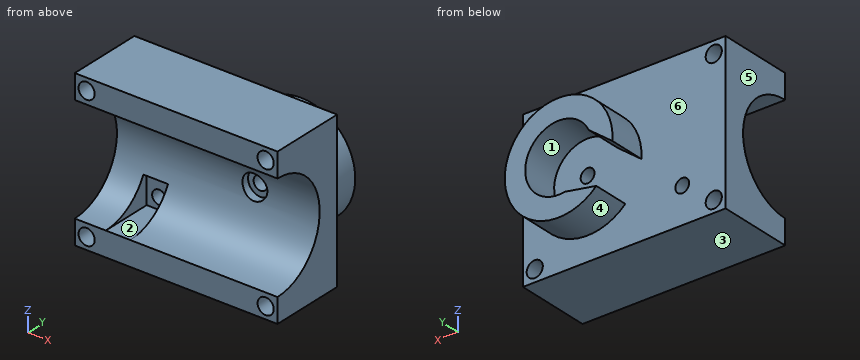
```python
from build123d import *

# Parameters (mm, degrees)
SKETCH1_W           = 60
SKETCH1_H           = 36
BOSS_EXTRUDE1_DEPTH = 35
SKETCH3_R           = 12.375
CUT_EXTRUDE1_DEPTH  = 61
SKETCH5_R           = 1.875
CUT_EXTRUDE2_DEPTH  = 40
CUT_EXTRUDE3_START  = 30
SKETCH7_W           = 36
SKETCH7_H           = 17.5
CUT_EXTRUDE3_DEPTH  = 61
SKETCH19_R          = 2.885
CUT_EXTRUDE13_DEPTH = 14
SKETCH20_R          = 1.6
CUT_EXTRUDE14_DEPTH = 13
SKETCH21_R          = 1.6
CUT_EXTRUDE15_DEPTH = 18.5000001
SKETCH22_W          = 5.7
SKETCH22_H          = 6.805143355
CUT_EXTRUDE16_DEPTH = 12
SKETCH23_R          = 12.5
SKETCH23_R_2        = 7.75
BOSS_EXTRUDE2_DEPTH = 8.5
CUT_EXTRUDE17_DEPTH = 8.5
SKETCH25_W          = 40.384912637
SKETCH25_H          = 20.483413903
CUT_EXTRUDE18_DEPTH = 13


with BuildPart() as part:
    # Sketch1 → Boss-Extrude1 (new body)
    with BuildSketch(Plane(origin=(0, 0, 0), x_dir=(1, 0, 0), z_dir=(0, 1, 0))):
        Rectangle(SKETCH1_W, SKETCH1_H)
    extrude(amount=BOSS_EXTRUDE1_DEPTH)

    # Sketch3 → Cut-Extrude1 (cut, through all)
    with BuildSketch(Plane(origin=(30, 0, 0), x_dir=(0, 0, -1), z_dir=(1, 0, 0))):
        with Locations((0, 17.5)):
            Circle(SKETCH3_R)
    extrude(amount=-CUT_EXTRUDE1_DEPTH, mode=Mode.SUBTRACT)

    # Sketch5 → Cut-Extrude2 (cut)
    with BuildSketch(Plane(origin=(0, 35, 0), x_dir=(1, 0, 0), z_dir=(0, 1, 0))):
        with Locations((27.25, -15.25)):
            Circle(SKETCH5_R)
        with Locations((27.25, 15.25)):
            Circle(SKETCH5_R)
        with Locations((-14.25, -15.25)):
            Circle(SKETCH5_R)
        with Locations((-14.25, 15.25)):
            Circle(SKETCH5_R)
    extrude(amount=-CUT_EXTRUDE2_DEPTH, mode=Mode.SUBTRACT)

    # Sketch7 → Cut-Extrude3 (cut, through all)
    with BuildSketch(Plane(origin=(0, 0, 0), x_dir=(0, 0, -1), z_dir=(1, 0, 0)).offset(CUT_EXTRUDE3_START)):
        with Locations((0, 8.75)):
            Rectangle(SKETCH7_W, SKETCH7_H)
    extrude(amount=-CUT_EXTRUDE3_DEPTH, mode=Mode.SUBTRACT)

    # Sketch19 → Cut-Extrude13 (cut)
    with BuildSketch(Plane.XZ.offset(-17.5)):
        with Locations((15, 0)):
            Circle(SKETCH19_R)
    extrude(amount=-CUT_EXTRUDE13_DEPTH, mode=Mode.SUBTRACT)

    # Sketch20 → Cut-Extrude14 (cut)
    with BuildSketch(Plane.XZ.offset(-31.5)):
        with Locations((15, 0)):
            Circle(SKETCH20_R)
    extrude(amount=-CUT_EXTRUDE14_DEPTH, mode=Mode.SUBTRACT)

    # Sketch21 → Cut-Extrude15 (cut, through all)
    with BuildSketch(Plane(origin=(0, 35, 0), x_dir=(1, 0, 0), z_dir=(0, 1, 0))):
        with Locations((-6.937800687, 9.733082811)):
            Circle(SKETCH21_R)
    extrude(amount=-CUT_EXTRUDE15_DEPTH, mode=Mode.SUBTRACT)

    # Sketch22 → Cut-Extrude16 (cut)
    with BuildSketch(Plane.XZ.offset(-17.5)):
        with Locations((-6.954606202, -8.972428323)):
            Rectangle(SKETCH22_W, SKETCH22_H)
    extrude(amount=-CUT_EXTRUDE16_DEPTH, mode=Mode.SUBTRACT)

    # Sketch23 → Boss-Extrude2 (add)
    with BuildSketch(Plane(origin=(0, 35, 0), x_dir=(1, 0, 0), z_dir=(0, 1, 0))):
        with Locations((15, 0)):
            Circle(SKETCH23_R)
        with Locations((15, 0)):
            Circle(SKETCH23_R_2, mode=Mode.SUBTRACT)
    extrude(amount=BOSS_EXTRUDE2_DEPTH)

    # Sketch24 → Cut-Extrude17 (cut)
    with BuildSketch(Plane(origin=(0, 43.5, 0), x_dir=(1, 0, 0), z_dir=(0, 1, 0))):
        Polygon((-6.937800687, 8.133082811), (13.574185936, -7.617713191), (13.574185936, 7.617713191), (-6.317460524, 11.207931305), align=None)
    extrude(amount=-CUT_EXTRUDE17_DEPTH, mode=Mode.SUBTRACT)

    # Sketch25 → Cut-Extrude18 (cut)
    with BuildSketch(Plane.ZY.offset(30)):
        with Locations((-0.290957584, 25.898615679)):
            Rectangle(SKETCH25_W, SKETCH25_H)
    extrude(amount=-CUT_EXTRUDE18_DEPTH, mode=Mode.SUBTRACT)


solid = part.part
```
Model file for the job. Use its own axes, mm. Face numbers are marked on the shaded views. A direction names the side the tool comes from. Coordinates: 2 decimals unless noted, no trailing zeros. Loops run counter-clockwise (first coordinate to the right, second up) from the corner with the lowest first, then second, coordinate; pieces in that order, holes last. Notation, with made-up numbers: (31.5, 62.5) - (36.5, 62.5) arc R23 ccw to (36.5, 92.5) - close; hole circle Ø11 at (26, 83.25). An arc over 180 degrees is marked (long way). Write item = value, one per line. Start each with the question number.
Item 1: Saw through at C-C, the plane z = 16. List the corners of the cut face in (x, y).
Item 2: 3-axis set-ups, long thin cutter, end or side, ignore diameter. For the marked faces 5 and 6: which of +Z, -Z, +X, -X, +Y, -Y reach the whole face in a straight line?
Item 3: Saw through at B-B, the plane x = -14.25. List the corners of the cut face in (y, z) (3 decimals).
Item 4: Saw through at D-D, the plane y = 22.5. List the corners of the cut face in (x, z) (3 decimals), then the cut area to 3 significant figures.
Item 5: Pull direction X, two halves, no side cores. Call the marked faces 1, 2, 3 and 4: +X half, -X half, draft (parallel to the pull), parting line (faces both ways), or undercut.
Item 6: Saw through at A-A, the plane x = 15. List the corners of the cut face in (y, z) (3 decimals).
Item 7: Wall check: probe 1 along Z at (x, y) = (15, 37); probe 2 along Z at (x, y) = (15, 30.75) (3 decimals); probe 3 along Z at (x, y) = (-14.25, 27) (3 decimals). Give the ranges that are in metal, low to high. Write a range as [from, to].
Item 8: Drop flat-ended pins along their axis: pin 1 Ø4 at (y, z) = (39.5, 11) entering from -X; pin 2 Ø9.5 at (x, z) = (15, 0) entering from +Y; pin 3 Ø3 at (x, z) = (15, -1) entering from -Y. Give the stop position or say it passes through.
Answers:
q1.outline = (-17, 17.5) - (-15.97, 17.5) - (-15.97, 35) - (-17, 35) - close; (-12.53, 17.5) - (25.53, 17.5) - (25.53, 35) - (-12.53, 35) - close; (28.97, 17.5) - (30, 17.5) - (30, 35) - (28.97, 35) - close
q2.face_5 = +Z, -Z, -X, +Y, -Y
q2.face_6 = +Y
q3.outline = (17.5, -18) - (35, -18) - (35, -17.125) - (17.5, -17.125) - close; (17.5, -13.375) - (35, -13.375) - (35, 13.375) - (17.5, 13.375) - (17.5, 12.375) arc R12.375 cw to (17.5, -12.375) - close; (17.5, 17.125) - (35, 17.125) - (35, 18) - (17.5, 18) - close
q4.outline = (-17, -18) - (30, -18) - (30, -11.32) - (-4.105, -11.32) - (-4.105, -12.375) - (-9.805, -12.375) - (-9.805, -11.32) - (-17, -11.32) - close; (-17, 11.32) - (30, 11.32) - (30, 18) - (-17, 18) - close; hole circle Ø3.75 at (-14.25, -15.25); hole circle Ø3.75 at (-14.25, 15.25); hole circle Ø3.75 at (27.25, -15.25); hole circle Ø3.75 at (27.25, 15.25)
q4.area = 578 mm2
q5.face_1 = undercut
q5.face_2 = undercut
q5.face_3 = draft
q5.face_4 = parting line
q6.outline = (17.5, -18) - (35, -18) - (35, -12.5) - (43.5, -12.5) - (43.5, -7.75) - (35, -7.75) - (35, -1.6) - (31.5, -1.6) - (31.5, -2.885) - (29.534, -2.885) arc R12.375 cw to (17.5, -12.375) - close; (17.5, 12.375) arc R12.375 cw to (29.534, 2.885) - (31.5, 2.885) - (31.5, 1.6) - (35, 1.6) - (35, 7.75) - (43.5, 7.75) - (43.5, 12.5) - (35, 12.5) - (35, 18) - (17.5, 18) - close
q7.probe_1 = [-12.5, -7.75], [7.75, 12.5]
q7.probe_2 = [-18, -2.885], [2.885, 18]
q7.probe_3 = [-18, -17.125], [-13.375, -7.93], [7.93, 13.375], [17.125, 18]
q8.pin_1 = 6.33
q8.pin_2 = 35
q8.pin_3 = 31.5
